```python
from build123d import *

# Parameters (mm, degrees)
CROQUIS3_R                  = 3
CORTAR_EXTRUIR1_DEPTH       = 21.184253764
TALADRO_ROSCADO_4_403_D     = 2.2606
TALADRO_ROSCADO_4_404_D     = 2.2606
TALADRO_ROSCADO_4_404_DEPTH = 12.699
TALADRO_ROSCADO_4_404_TIP   = 0.679152758


with BuildPart() as part:
    # Croquis2 → Revolución1 (revolve)
    with BuildSketch(Plane(origin=(0, 0, 0), x_dir=(0, 0, -1), z_dir=(1, 0, 0))):
        Polygon((0, 0), (0, 6.035), (4.13, 6.035), (4.13, 12.7), (9.21, 12.7), (9.21, 0), align=None)
    revolve(axis=Axis((0, 0, -9.21), (0, 0, 1)))

    # Croquis3 → Cortar-Extruir1 (cut, through all)
    with BuildSketch(Plane.XY):
        Circle(CROQUIS3_R)
    extrude(amount=-CORTAR_EXTRUIR1_DEPTH, mode=Mode.SUBTRACT)

    # Taladro roscado #4-403 (through all)
    with Locations(Plane.XY.offset(-4.13)):
        with Locations((-9.53, 0), (-4.765, 8.253222098), (4.765, 8.253222098), (9.53, 0), (4.765, -8.253222098), (-4.765, -8.253222098), (0, 0)):
            Hole(TALADRO_ROSCADO_4_403_D / 2)

    # Taladro roscado #4-404
    with Locations(Plane(origin=(0, 12.7, 0), x_dir=(1, 0, 0), z_dir=(0, 1, 0))):
        with Locations((0, 6.67), (0, 2.5)):
            Hole(TALADRO_ROSCADO_4_404_D / 2, depth=TALADRO_ROSCADO_4_404_DEPTH)
            with Locations((0, 0, -(TALADRO_ROSCADO_4_404_DEPTH + TALADRO_ROSCADO_4_404_TIP / 2))):  # 118° drill point
                Cone(0, TALADRO_ROSCADO_4_404_D / 2, TALADRO_ROSCADO_4_404_TIP, mode=Mode.SUBTRACT)


solid = part.part
```
Geometry: final body of the model. Coordinates: model frame, mm. A direction names the side the tool comes from. Round coordinates to 2 decimals unless told otherwise and drop trailing zeros. Loops run counter-clockwise (first coordinate to the right, second up) from the corner with the lowest first, then second, coordinate; pieces in that order, holes last. Notation, with made-up numbers: (13.25, -38) -> (54.25, -38) arc R24 ccw to (54.25, 1) -> close; hole circle Ø2 at (-33, -39). An arc over 180 degrees is marked (long way). Use one line per item in the form item = value.
Item 1: Cut plane D-D on z = -7.5. Output: boundary loops of the cut face in (x, y) (3 decimals).
Evaluation:
outline = (-0.767, 2.9) -> (-0.767, 12.677) arc R12.7 ccw (long way) to (0.767, 12.677) -> (0.767, 2.9) arc R3 cw (long way) to start; hole circle Ø2.261 at (-9.53, 0); hole circle Ø2.261 at (-4.765, -8.253); hole circle Ø2.261 at (-4.765, 8.253); hole circle Ø2.261 at (4.765, -8.253); hole circle Ø2.261 at (4.765, 8.253); hole circle Ø2.261 at (9.53, 0)
Item 2: Cut plane A-A on x = 0. Output: boundary loops of the cut face in (y, z) (3 decimals).
Evaluation:
outline = (-12.7, -9.21) -> (-3, -9.21) -> (-3, 0) -> (-6.035, 0) -> (-6.035, -4.13) -> (-12.7, -4.13) -> close; (3, -9.21) -> (12.7, -9.21) -> (12.7, -7.8) -> (3, -7.8) -> close; (3, -5.54) -> (12.7, -5.54) -> (12.7, -4.13) -> (6.035, -4.13) -> (6.035, -3.63) -> (3, -3.63) -> close; (3, -1.37) -> (6.035, -1.37) -> (6.035, 0) -> (3, 0) -> close
Item 3: Contact query for flat-ended pins moving along their axis: pin 1 Ø1.4 at (x, y) = (-4.76, -8.25) entering from -Z; pin 2 Ø2 at (y, z) = (7, -7.5) entering from +X; pin 3 Ø2 at (x, z) = (8.5, -3.5) entering from +Y; pin 4 Ø10 at (x, y) = (10, -8) entering from +Z. Output: stop coordinate, or through.
Evaluation:
pin_1 = through
pin_2 = 11.19
pin_3 = 10.08
pin_4 = -4.13
Item 4: Cut plane B-B on y = 0. Output: boundary loops of the cut face in (x, z) (3 decimals), then the cut area to 3 significant figures.
Evaluation:
outline = (-12.7, -9.21) -> (-10.66, -9.21) -> (-10.66, -4.13) -> (-12.7, -4.13) -> close; (-8.4, -9.21) -> (-3, -9.21) -> (-3, 0) -> (-6.035, 0) -> (-6.035, -4.13) -> (-8.4, -4.13) -> close; (3, -9.21) -> (8.4, -9.21) -> (8.4, -4.13) -> (6.035, -4.13) -> (6.035, 0) -> (3, 0) -> close; (10.66, -9.21) -> (12.7, -9.21) -> (12.7, -4.13) -> (10.66, -4.13) -> close
area = 101 mm2
Item 5: Access query for faces 5 (the flat face through (3, 3, -9.21)), 6 (the cylindrical face through (1.13, 4.38, -2.55)), 7 (the cylindrical face through (5.89, -1.31, -2.09)). Directions: +Z, -Z, +X, -X, +Y, -Y. A direction counts if a zero-diameter tool reaches every point of the face in a straight line with its end or side. Return the directions, or none.
Evaluation:
face_5 = -Z, +X, -X, +Y, -Y
face_6 = +Y
face_7 = +Z
Item 6: Material intervals for probe 1 along Z at (x, y) = (0, 9.25); probe 2 along Z at (x, y) = (0, 4.5); probe 3 along X at (y, z) = (-8.25, -6.75), sorted ascending.
Evaluation:
probe_1 = -9.21 to -7.8, -5.54 to -4.13
probe_2 = -9.21 to -7.8, -5.54 to -3.63, -1.37 to 0
probe_3 = -9.66 to -5.9, -3.63 to 3.63, 5.9 to 9.66
Item 7: Cut plane C-C on x = 9.53. Output: boundary loops of the cut face in (y, z).
Evaluation:
outline = (-8.39, -9.21) -> (-1.13, -9.21) -> (-1.13, -4.13) -> (-8.39, -4.13) -> close; (1.13, -9.21) -> (8.39, -9.21) -> (8.39, -4.13) -> (1.13, -4.13) -> close
Item 8: Draft query along X for faces 1 (the flat face through (5.5, 3, -4.13)), 2 (the cylindrical face through (-9, 1, -7)), 3 (the cylindrical face through (12.4, -2.75, -6.71)), 4 (the cylindrical face through (0.15, 7.67, -7.79)). Return one class per face: released by +X, released by -X, zero draft, split by the parting line, or undercut.
Evaluation:
face_1 = zero draft
face_2 = undercut
face_3 = split by the parting line
face_4 = undercut
